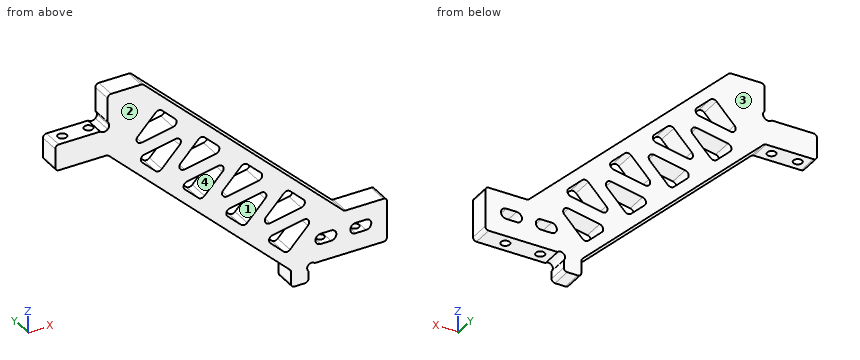
from build123d import *

# Parameters (mm, degrees)
EXTRUDE_1_DEPTH     = 3
FILLET_2_R          = 1
CUT_EXTRUDE_1_DEPTH = 6
FILLET_3_R          = 1.25
SKETCH_6_R          = 1.25
CUT_EXTRUDE_4_DEPTH = 108.570906848
SKETCH_7_R          = 1.25
CUT_EXTRUDE_5_DEPTH = 8


with BuildPart() as part:
    # ｽｹｯﾁ1 → ﾎﾞｽ - 押し出し1 (new, symmetric)
    with BuildSketch(Plane(origin=(0, 0, 0), x_dir=(1, 0, 0), z_dir=(0, 1, 0))):
        with BuildLine():
            Line((7.5, -2.121320344), (7.5, -10))
            Line((7.5, -10), (17.5, -10))
            Line((17.5, -10), (75.25, 45))
            Line((75.25, 45), (87.5, 45))
            Line((87.5, 45), (87.5, 57.5))
            Line((87.5, 57.5), (66.767766953, 57.5))
            ThreePointArc((66.767766953, 57.5), (65.883883476, 57.133883476), (65, 57.5))
            ThreePointArc((65, 57.5), (64.633883476, 58.383883476), (65, 59.267766953))
            Line((65, 59.267766953), (65, 62.5))
            Line((65, 62.5), (60, 62.5))
            Line((60, 62.5), (60, 57.5))
            Line((60, 57.5), (7.5, 7.5))
            Line((7.5, 7.5), (-7.5, 7.5))
            Line((-7.5, 7.5), (-7.5, 0))
            Line((-7.5, 0), (5.378679656, 0))
            ThreePointArc((5.378679656, 0), (6.439339828, 0.439339828), (7.5, 0))
            ThreePointArc((7.5, 0), (7.825159127, -0.486635023), (7.939339828, -1.060660172))
            ThreePointArc((7.939339828, -1.060660172), (7.825159127, -1.63468532), (7.5, -2.121320344))
        make_face()
        with BuildLine():
            ThreePointArc((68.5, 49.5), (67, 51), (68.5, 52.5))
            Line((68.5, 52.5), (71.5, 52.5))
            ThreePointArc((71.5, 52.5), (73, 51), (71.5, 49.5))
            Line((71.5, 49.5), (68.5, 49.5))
        make_face(mode=Mode.SUBTRACT)
        with BuildLine():
            ThreePointArc((78.5, 49.5), (77, 51), (78.5, 52.5))
            Line((78.5, 52.5), (81.5, 52.5))
            ThreePointArc((81.5, 52.5), (83, 51), (81.5, 49.5))
            Line((81.5, 49.5), (78.5, 49.5))
        make_face(mode=Mode.SUBTRACT)
    extrude(amount=EXTRUDE_1_DEPTH, both=True)

    # ﾌｨﾚｯﾄ2
    fillet_2_edges = [part.edges().sort_by_distance(p)[0] for p in [
        (87.5, -1.5, -57.5),
        (87.5, -1.5, -45),
        (75.25, -1.5, -45),
        (17.5, -1.5, 10),
        (7.5, -1.5, 10),
        (-7.5, -1.5, 0),
        (-7.5, -1.5, -7.5),
        (7.5, -1.5, -7.5),
        (60, -1.5, -57.5),
        (60, -1.5, -62.5),
        (65, -1.5, -62.5),
    ]]
    fillet(fillet_2_edges, radius=FILLET_2_R)

    # ｽｹｯﾁ2 → ｶｯﾄ - 押し出し1 (cut)
    with BuildSketch(Plane(origin=(0, 3, 0), x_dir=(1, 0, 0), z_dir=(0, 1, 0))):
        Polygon((58.862068966, 52.273399015), (52.344827586, 46.066502463), (67.530321046, 43.17173433), align=None)
        Polygon((50.171921182, 42.616115412), (65.357414642, 39.721347279), (58.840173263, 33.514450727), align=None)
        Polygon((46.619704433, 40.614004222), (40.102463054, 34.407107671), (55.287956514, 31.512339537), align=None)
        Polygon((37.92955665, 30.956720619), (53.11505011, 28.061952486), (46.597808731, 21.855055934), align=None)
        Polygon((34.377339901, 28.95460943), (27.860098522, 22.747712878), (43.045591982, 19.852944745), align=None)
        Polygon((25.687192118, 19.297325827), (40.872685578, 16.402557694), (34.355444199, 10.195661142), align=None)
        Polygon((22.134975369, 17.295214638), (15.61773399, 11.088318086), (30.80322745, 8.193549953), align=None)
        Polygon((13.444827586, 7.637931034), (28.630321046, 4.743162901), (22.113079667, -1.46373365), align=None)
    extrude(amount=-CUT_EXTRUDE_1_DEPTH, mode=Mode.SUBTRACT)

    # ﾌｨﾚｯﾄ3
    fillet_3_edges = [part.edges().sort_by_distance(p)[0] for p in [
        (58.862068966, 0, -52.273399015),
        (67.530321046, 0, -43.17173433),
        (52.344827586, 0, -46.066502463),
        (46.619704433, 0, -40.614004222),
        (55.287956514, 0, -31.512339537),
        (40.102463054, 0, -34.407107671),
        (58.840173263, 0, -33.514450727),
        (50.171921182, 0, -42.616115412),
        (65.357414642, 0, -39.721347279),
        (34.377339901, 0, -28.95460943),
        (43.045591982, 0, -19.852944745),
        (27.860098522, 0, -22.747712878),
        (46.597808731, 0, -21.855055934),
        (37.92955665, 0, -30.956720619),
        (53.11505011, 0, -28.061952486),
        (22.134975369, 0, -17.295214638),
        (30.80322745, 0, -8.193549953),
        (15.61773399, 0, -11.088318086),
        (34.355444199, 0, -10.195661142),
        (25.687192118, 0, -19.297325827),
        (40.872685578, 0, -16.402557694),
        (22.113079667, 0, 1.46373365),
        (13.444827586, 0, -7.637931034),
        (28.630321046, 0, -4.743162901),
    ]]
    fillet(fillet_3_edges, radius=FILLET_3_R)

    # ｽｹｯﾁ6 → ｶｯﾄ - 押し出し4 (cut, through all)
    with BuildSketch(Plane.XY):
        with Locations((-3.75, 0)):
            Circle(SKETCH_6_R)
        with Locations(Location((3.75, 0, 0), (0, 0, 180))):
            Circle(SKETCH_6_R)
    extrude(amount=-CUT_EXTRUDE_4_DEPTH, mode=Mode.SUBTRACT)

    # ｽｹｯﾁ7 → ｶｯﾄ - 押し出し5 (cut)
    with BuildSketch(Plane(origin=(0, 0, -57.5), x_dir=(-1, 0, 0), z_dir=(0, 0, -1))):
        with Locations((-70, 0)):
            Circle(SKETCH_7_R)
        with Locations((-80, 0)):
            Circle(SKETCH_7_R)
    extrude(amount=-CUT_EXTRUDE_5_DEPTH, mode=Mode.SUBTRACT)


solid = part.part
Verification items for the finished model (mm, model axes). Face numbers are marked on the shaded views. A direction names the side the tool comes from. Give positions to 0.01 mm unless a question says otherwise; leave off trailing zeros. Loops run counter-clockwise (first coordinate to the right, second up) from the corner with the lowest first, then second, coordinate; pieces in that order, holes last.
1) Draft check along X on the marked faces 1 and 2. Enter one of: pulls with the +X half, pulls with the -X half, needs draft (parallel to the pull), parting line crosses it, or undercut.
2) Depth check by flat-ended pin: pin 1 Ø1.5 at (x, y) = (56, 2.5) entering from +Z; pin 2 Ø4 at (x, z) = (56, -54.5) entering from +Y; pin 3 Ø1.8 at (y, z) = (-1, -60.5) entering from +X; pin 4 Ø2 at (x, y) = (-3.75, 0) entering from +Z. Enter the tip coordinate at first touch or a pass-through.
3) Sectioned sample at A-A, the plane x = 80. Enter the section's corners in (y, z), then the cut area to 3 significant figures.
4) Sectioned sample at B-B, the plane x = 3.75. Enter the section's corners in (y, z).
5) Set-up check for the marked faces 3 and 4: record each of +Z, -Z, +X, -X, +Y, -Y from which the full face is reachable in a straight line by a thin tool's end or side.
6) Sectioned sample at C-C, the plane x = 70. Enter the section's corners in (y, z), then the cut area to 3 significant figures.
7) Thickness scan on line 1 along Y through (x, z) = (3.75, -1.75); line 2 along X through (y, z) = (-0.15, -54) (3 decimals); line 3 along X through (y, z) = (-0.7, -39.5) (3 decimals). Record the ranges inside material, lowest first.
Answers:
1. face 1: undercut
1. face 2: needs draft
2. pin 1: stops at z = -25.95
2. pin 2: stops at y = 3
2. pin 3: stops at x = 65
2. pin 4: passes through
3. outline: (-3, -57.5) - (-1.25, -57.5) - (-1.25, -52.5) - (-3, -52.5) - close; (-3, -49.5) - (3, -49.5) - (3, -45) - (-3, -45) - close; (1.25, -57.5) - (3, -57.5) - (3, -52.5) - (1.25, -52.5) - close
3. area: 44.5 mm2
4. outline: (-3, -7.5) - (-1.25, -7.5) - (-1.25, 0) - (-3, 0) - close; (1.25, -7.5) - (3, -7.5) - (3, 0) - (1.25, 0) - close
5. face 3: +Z, -Z, +X, -X, +Y
5. face 4: +Y, -Y
6. outline: (-3, -57.5) - (-1.25, -57.5) - (-1.25, -52.5) - (-3, -52.5) - close; (-3, -49.5) - (3, -49.5) - (3, -40) - (-3, -40) - close; (1.25, -57.5) - (3, -57.5) - (3, -52.5) - (1.25, -52.5) - close
6. area: 74.5 mm2
7. line 1: y = -3 to -1.25, 1.25 to 3
7. line 2: x = 56.325 to 68.759, 71.241 to 78.759, 81.241 to 87.5
7. line 3: x = 41.1 to 45.45, 47.681 to 53.14, 63.856 to 69.475
